Part model, mm, in its own coordinate system. Face numbers are marked on the shaded views. A direction names the side the tool comes from. Coordinates: 2 decimals unless noted, no trailing zeros. Write each loop counter-clockwise with the first axis right and the second up, starting at its lowest first coordinate (ties: lowest second). Pieces come first, ordered by that corner, then holes. Notation, with made-up numbers: (32.25, 86.5) -> (75.25, 86.5) arc R23 ccw to (75.25, 113.5) -> close; hole circle Ø9 at (82, 21.25). An arc over 180 degrees is marked (long way). Write item = value, one per line. Start each with the question number.
Q1. Probe line 1 (Y direction, x = 0, z = 210); line 2 (Y direction, x = 0, z = 40). List the from-to ranges inside material, lowest first.
Q2. Band-saw the part on B-B, the plane z = 168. List the corners of the cut face in (x, y), plus the area to 3 significant figures.
Q3. Tool access for the marked faces 1 and 2: list every direction of +Z, -Z, +X, -X, +Y, -Y with a clear straight run to the whole face (end or side of a thin tool).
Q4. Pin check, flat tips, straight feed: P1, Ø1, axis at x = -19.5, z = 175.5, coming from the +Y side; P2, Ø3, axis at x = -10, z = 197.5, coming from the -Y side; P3, Ø6, axis at y = -10, z = 168, coming from the +X side; P4, Ø8, axis at x = -23, y = -35, coming from the -Z side. Stop position of each tip, or through.
Q5. Pull direction Y, two halves, no side cores. Call the marked faces 3 and 4: released by +Y, released by -Y, zero draft, split by the parting line, or undercut.
Q6. Band-saw the part on A-A, the plane x = 0. List the corners of the cut face in (y, z) (3 decimals).
Q7. Band-saw the part on D-D, the plane z = 202. List the corners of the cut face in (x, y), plus the area to 3 significant figures.
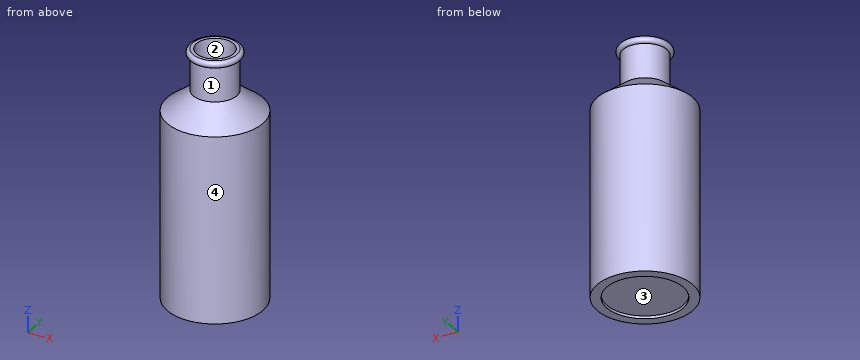
from build123d import *


with BuildPart() as f1:
    # F0 (on Front) → F1 (revolve)
    with BuildSketch(Plane.XZ):
        with BuildLine():
            Line((35.56, 0), (44.45, 0))
            Line((44.45, 0), (44.45, 172.72))
            Line((44.45, 172.72), (20.32, 191.77))
            Line((20.32, 191.77), (20.32, 223.52))
            ThreePointArc((20.32, 223.52), (23.495, 226.695), (20.32, 229.87))
            Line((20.32, 229.87), (17.272, 229.87))
            Line((17.272, 229.87), (17.272, 226.822))
            Line((17.272, 226.822), (17.272, 190.292933))
            Line((17.272, 190.292933), (41.402, 171.242933))
            Line((41.402, 171.242933), (41.402, 5.588))
            Line((41.402, 5.588), (0, 5.588))
            Line((0, 5.588), (0, 2.54))
            Line((0, 2.54), (35.56, 2.54))
            Line((35.56, 2.54), (35.56, 0))
        make_face()
    revolve(axis=Axis((0, 0, 114.935), (0, 0, -1)))


solid = f1.part
Ans:
q1.line_1 = -20.32 to -17.27, 17.27 to 20.32
q1.line_2 = -44.45 to -41.4, 41.4 to 44.45
q2.outline = circle Ø88.9 at (0, 0); hole circle Ø82.8 at (0, 0)
q2.area = 822 mm2
q3.face_1 = none
q3.face_2 = +Z
q4.P1 = 36.75
q4.P2 = -18.46
q4.P3 = 43.9
q4.P4 = 0
q5.face_3 = undercut
q5.face_4 = split by the parting line
q6.outline = (-44.45, 0) -> (-35.56, 0) -> (-35.56, 2.54) -> (35.56, 2.54) -> (35.56, 0) -> (44.45, 0) -> (44.45, 172.72) -> (20.32, 191.77) -> (20.32, 223.52) arc R3.175 ccw to (20.32, 229.87) -> (17.272, 229.87) -> (17.272, 190.293) -> (41.402, 171.243) -> (41.402, 5.588) -> (-41.402, 5.588) -> (-41.402, 171.243) -> (-17.272, 190.293) -> (-17.272, 229.87) -> (-20.32, 229.87) arc R3.175 ccw to (-20.32, 223.52) -> (-20.32, 191.77) -> (-44.45, 172.72) -> close
q7.outline = circle Ø40.64 at (0, 0); hole circle Ø34.54 at (0, 0)
q7.area = 360 mm2
